```python
from build123d import *

# Parameters (mm, degrees)
SKETCH1_R           = 25
BOSS_EXTRUDE1_DEPTH = 40
CUT_EXTRUDE1_START  = -10
CUT_EXTRUDE1_DEPTH  = 10
CIRPATTERN1_COUNT   = 3
SKETCH7_R           = 15.1
CUT_EXTRUDE3_DEPTH  = 8.7


with BuildPart() as part:
    # Sketch1 → Boss-Extrude1 (new body)
    with BuildSketch(Plane(origin=(0, 0, 0), x_dir=(1, 0, 0), z_dir=(0, 1, 0))):
        with Locations(Location((0, 0, 0), (0, 0, 270))):
            Circle(SKETCH1_R)
    extrude(amount=BOSS_EXTRUDE1_DEPTH)

    # Sketch2 → Cut-Extrude1 (cut)
    with BuildSketch(Plane(origin=(0, 40, 0), x_dir=(1, 0, 0), z_dir=(0, 1, 0)).offset(CUT_EXTRUDE1_START)):
        with BuildLine():
            Line((-25, 0), (-2, 0))
            Line((-2, 0), (-2, -20.4))
            Line((-2, -20.4), (-12.2, -20.4))
            Line((-12.2, -20.4), (-12.2, -10.2))
            Line((-12.2, -10.2), (-22.824548188, -10.2))
            ThreePointArc((-22.824548188, -10.2), (-24.450089005, -5.214704943), (-25, 0))
        make_face()
    cut_extrude1 = extrude(amount=CUT_EXTRUDE1_DEPTH, mode=Mode.SUBTRACT)

    # CirPattern1: Cut-Extrude1 ×3 about axis
    cirpattern1_axis = Axis((0, 0, 0), (0, 1, 0))
    for i in range(1, CIRPATTERN1_COUNT):
        add(cut_extrude1.rotate(cirpattern1_axis, i * 360 / CIRPATTERN1_COUNT), mode=Mode.SUBTRACT)

    # Sketch7 → Cut-Extrude3 (cut)
    with BuildSketch(Plane.XZ):
        with Locations(Location((0, 0, 0), (0, 0, 270))):
            Circle(SKETCH7_R)
    extrude(amount=-CUT_EXTRUDE3_DEPTH, mode=Mode.SUBTRACT)


solid = part.part
```
Geometry: final body of the model. Coordinates: model frame, mm. A direction names the side the tool comes from. Round coordinates to 2 decimals unless told otherwise and drop trailing zeros. Order: outer loops, then holes, each group sorted by start corner. A loop starts at its lowest first (then second) coordinate and runs counter-clockwise, first axis right, second up. Notation, with made-up numbers: M -27,32.5 L 32,32.5 A11 cw 32,48.5 Z; hole C 24.5,-31.5 d3. An arc over 180 degrees is marked long. Use one line per item in the form item = value. Start each with the question number.
Q1. Cut plane C-C (x = -5). Return loops of the section in (y, z).
Q2. Mould query, pull axis X, two halves, no side actions, for faces 6 (the face through (7.509, 19.72, 23.846)), 7 (the face through (0, 40, 0)), 8 (the face through (-7, 35, 20.4)). Classes: +X half, -X half, draft (parallel to the pull), parting line (faces both ways), or undercut.
Q3. Access query for faces 1 (the face through (0, 8.7, 0)), 2 (the face through (-17, 35, 10.2)), 3 (the face through (19.41, 34.93, 2.88)), 4 (the face through (-11, 0, 11)), 5 (the face through (17.55, 34.93, 10)). Directions: +Z, -Z, +X, -X, +Y, -Y. A direction counts if a zero-diameter tool reaches every point of the face in a straight line with its end or side. Return the directions, or none.
Q4. Cut plane D-D (z = 16.5). Return loops of the section in (x, y), and give its area (3 significant figures).
Q5. Material intervals for line 1 (X direction, y = 5, z = 0); line 2 (X direction, y = 36, z = -17.5); line 3 (Y direction, x = 10, z = 11), sorted ascending. Write a range as [from, to].
Q6. Cut plane B-B (z = -5.5). Return loops of the section in (x, y), and give its area (3 significant figures).
Q7. Pin query (flat end, axial travel): pin 1 Ø3 at (x, y) = (-5, 36) entering from -Z; pin 2 Ø1.5 at (x, y) = (-14.5, 13) entering from -Z; pin 3 Ø4 at (x, y) = (-13.5, 26.5) entering from +Z. Return the tip coordinate at first contact, or that it passes through.
Q8. Cut plane A-A (y = 34.5). Return loops of the section in (x, z), and give its area (3 significant figures).
Geometry results:
q1.outline = M 0,-24.49 L 40,-24.49 L 40,-16.97 L 30,-16.97 L 30,-5.2 L 40,-5.2 L 40,0 L 30,0 L 30,20.4 L 40,20.4 L 40,24.49 L 0,24.49 L 0,14.25 L 8.7,14.25 L 8.7,-14.25 L 0,-14.25 Z
q2.face_6 = parting line
q2.face_7 = draft
q2.face_8 = undercut
q3.face_1 = -Y
q3.face_2 = -X, +Y
q3.face_3 = +Y
q3.face_4 = +Z, -Z, +X, -X, -Y
q3.face_5 = +Z, +Y
q4.outline = M -18.78,0 L 18.78,0 L 18.78,30 L 9.53,30 L 9.53,40 L -2,40 L -2,30 L -12.2,30 L -12.2,40 L -18.78,40 Z
q4.area = 1,310 mm^2
q5.line_1 = [-25, -15.1], [15.1, 25]
q5.line_2 = [-17.85, -13.45], [-5.91, -1.67], [10.1, 17.85]
q5.line_3 = [8.7, 30]
q6.outline = M -24.39,0 L -14.06,0 L -14.06,8.7 L 14.06,8.7 L 14.06,0 L 24.39,0 L 24.39,40 L 20.38,40 L 20.38,30 L 13.53,30 L 13.53,40 L 3.18,40 L 3.18,30 L -5.53,30 L -5.53,40 L -24.39,40 Z
q6.area = 1,550 mm^2
q7.pin_1 = -24.75
q7.pin_2 = -20.88
q7.pin_3 = 22.2
q8.outline = M -25,0 A25 ccw 2.58,-24.87 L -2.73,-15.67 L -11.57,-20.77 L -16.67,-11.93 L 1,-1.73 L 12.5,-21.65 A25 ccw 20.25,14.67 L 14.93,5.47 L 23.77,0.37 L 18.67,-8.47 L 1,1.73 L 12.5,21.65 A25 ccw -22.82,10.2 L -12.2,10.2 L -12.2,20.4 L -2,20.4 L -2,0 Z
q8.area = 969 mm^2
